Build history of the part. All positions in model axes, mm. Coordinates: 2 decimals unless noted, no trailing zeros. Order: outer loops, then holes, each group sorted by start corner. A loop starts at its lowest first (then second) coordinate and runs counter-clockwise, first axis right, second up. Notation, with made-up numbers: (17, 86.5) - (61, 86.5) arc R29 ccw to (61, 121.5) - close; hole circle Ø1 at (20.25, 72). An arc over 180 degrees is marked (long way). Return JSON: item names as keys, results as strings.
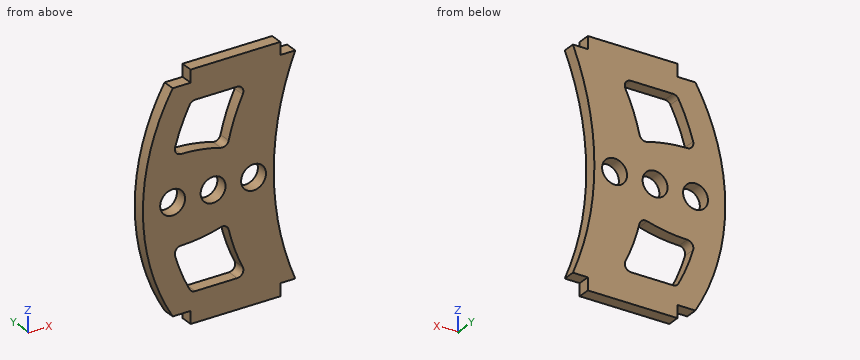
from build123d import *

# Parameters (mm, degrees)
SKETCH2_R           = 2
BOSS_EXTRUDE1_DEPTH = 2


with BuildPart() as part:
    # Sketch2 → Boss-Extrude1 (new body)
    with BuildSketch(Plane(origin=(0, 0, 0), x_dir=(1, 0, 0), z_dir=(0, 1, 0))):
        with BuildLine():
            Line((7.961413572, 38.398358915), (10.842933693, 38.398358915))
            Line((10.842933693, 38.398358915), (10.842933693, 40.398358915))
            Line((10.842933693, 40.398358915), (25.242933693, 40.398358915))
            Line((25.242933693, 40.398358915), (25.242933693, 38.398358915))
            Line((25.242933693, 38.398358915), (27.643012608, 38.398358915))
            ThreePointArc((27.643012608, 38.398358915), (24.192745703, 20.998358915), (27.643012608, 3.598358915))
            Line((27.643012608, 3.598358915), (25.242933693, 3.598358915))
            Line((25.242933693, 3.598358915), (25.242933693, 1.598358915))
            Line((25.242933693, 1.598358915), (10.842933693, 1.598358915))
            Line((10.842933693, 1.598358915), (10.842933693, 3.598358915))
            Line((10.842933693, 3.598358915), (7.961413572, 3.598358915))
            ThreePointArc((7.961413572, 3.598358915), (3.171685738, 20.998358915), (7.961413572, 38.398358915))
        make_face()
        with Locations(Location((14.44517784, 20.998358915, 0), (0, 0, 270))):
            Circle(SKETCH2_R, mode=Mode.SUBTRACT)
        with Locations(Location((7.94517784, 20.998358915, 0), (0, 0, 270))):
            Circle(SKETCH2_R, mode=Mode.SUBTRACT)
        with Locations(Location((20.94517784, 20.998358915, 0), (0, 0, 270))):
            Circle(SKETCH2_R, mode=Mode.SUBTRACT)
        with BuildLine():
            Line((11.558407931, 6.398358915), (18.314191235, 6.398358915))
            ThreePointArc((18.314191235, 6.398358915), (19.162339122, 6.868599384), (19.21282009, 7.837068593))
            ThreePointArc((19.21282009, 7.837068593), (17.901234233, 10.95935639), (16.949906233, 14.209573857))
            ThreePointArc((16.949906233, 14.209573857), (16.483665754, 14.844744909), (15.702159941, 14.945099841))
            ThreePointArc((15.702159941, 14.945099841), (12.522935582, 14.264828801), (9.281614764, 14.011697267))
            ThreePointArc((9.281614764, 14.011697267), (8.491111108, 13.609072345), (8.331792637, 12.73636364))
            ThreePointArc((8.331792637, 12.73636364), (9.351564099, 9.771568101), (10.675191455, 6.929393398))
            ThreePointArc((10.675191455, 6.929393398), (11.04312428, 6.54133922), (11.558407931, 6.398358915))
        make_face(mode=Mode.SUBTRACT)
        with BuildLine():
            Line((11.558407931, 35.598358915), (18.314191235, 35.598358915))
            ThreePointArc((18.314191235, 35.598358915), (19.162339122, 35.128118447), (19.21282009, 34.159649238))
            ThreePointArc((19.21282009, 34.159649238), (17.901234233, 31.03736144), (16.949906233, 27.787143973))
            ThreePointArc((16.949906233, 27.787143973), (16.483665754, 27.151972922), (15.702159941, 27.05161799))
            ThreePointArc((15.702159941, 27.05161799), (12.522935582, 27.73188903), (9.281614764, 27.985020563))
            ThreePointArc((9.281614764, 27.985020563), (8.491111108, 28.387645486), (8.331792637, 29.26035419))
            ThreePointArc((8.331792637, 29.26035419), (9.351564099, 32.225149729), (10.675191455, 35.067324432))
            ThreePointArc((10.675191455, 35.067324432), (11.04312428, 35.455378611), (11.558407931, 35.598358915))
        make_face(mode=Mode.SUBTRACT)
    extrude(amount=BOSS_EXTRUDE1_DEPTH)


solid = part.part
1. Probe L1, parallel to X at y = 1.6, z = -22; L2, parallel to Z at x = 12.25, y = 0.4; L3, parallel to Z at x = 18.25, y = 1.6. List the from-to ranges inside material, lowest first.
Check values:
{"L1": "3.19 to 6.21, 9.68 to 12.71, 16.18 to 19.21, 22.68 to 24.2", "L2": "-40.4 to -35.6, -27.77 to -14.23, -6.4 to -1.6", "L3": "-40.4 to -35.6, -31.97 to -10.03, -6.4 to -1.6"}
2. Cut at A-A on z = -9.5. Give the cut face in (x, y) (3 decimals).
Check values:
{"outline": "(5.175, 0) - (9.463, 0) - (9.463, 2) - (5.175, 2) - close; (18.463, 0) - (25.666, 0) - (25.666, 2) - (18.463, 2) - close"}
3. Cut at D-D on z = -37. Give the cut face in (x, y), plus the area to 3 significant figures.
Check values:
{"outline": "(7.17, 0) - (27.09, 0) - (27.09, 2) - (7.17, 2) - close", "area": "39.8 mm²"}
4. Cut at C-C on y = 1.1. State how many separate pieces and enclosed holes the cut face has, plus the area to 3 significant figures.
Check values:
{"separate pieces": "1", "enclosed holes": "5", "area": "596 mm²"}
5. Cut at B-B on x = 17.75. Give the cut face in (y, z), plus the area to 3 significant figures.
Check values:
{"outline": "(0, -40.4) - (2, -40.4) - (2, -35.6) - (0, -35.6) - close; (0, -30.6) - (2, -30.6) - (2, -11.4) - (0, -11.4) - close; (0, -6.4) - (2, -6.4) - (2, -1.6) - (0, -1.6) - close", "area": "57.6 mm²"}
6. Drop flat-ended pins along their axis: pin 1 (2.5 mm diameter, centred on x = 14.45, z = -21, fed in from -Y); pin 2 (1 mm diameter, centred on x = 26.5, y = 0.5, fed in from -Z); pin 3 (1 mm diameter, centred on x = 9.5, y = 1.5, fed in from +Z). Give the stop position or say it passes through.
Check values:
{"pin 1": "through", "pin 2": "z = -38.4", "pin 3": "z = -3.6"}
